Model file for the job. Use its own axes, mm. A direction names the side the tool comes from. Coordinates: 2 decimals unless noted, no trailing zeros. Return JSON: item names as keys, results as strings.
```python
from build123d import *

# Parameters (mm, degrees)
F0_R     = 1
F1_DEPTH = 5
F3_DEPTH = 10.001
F4_R     = 0.3
F6_DEPTH = 2.54
F7_R     = 0.2


with BuildPart() as f1:
    # F0 (on Front) → F1 (new body, symmetric)
    with BuildSketch(Plane.XZ):
        with BuildLine():
            Line((-2, 2), (-2, 0))
            ThreePointArc((-2, 0), (0, -2), (2, 0))
            Line((2, 0), (2, 2))
            Line((2, 2), (0, 2))
            Line((0, 2), (-2, 2))
        make_face()
        Circle(F0_R, mode=Mode.SUBTRACT)
    extrude(amount=F1_DEPTH, both=True)

    # F2 (on face) → F3 (cut, through all)
    with BuildSketch(Plane.XZ.offset(5)):
        with BuildLine():
            Line((0.875, -1.7984368212), (0, 0))
            Line((0, 0), (-0.875, -1.7984368212))
            ThreePointArc((-0.875, -1.7984368212), (0, -2), (0.875, -1.7984368212))
        make_face()
    extrude(amount=-F3_DEPTH, mode=Mode.SUBTRACT)

    # F4
    f4_edges = [f1.edges().sort_by_distance(p)[0] for p in [
        (-0.875, 0, -1.798437),
        (0.875, 0, -1.798437),
        (-1.695582, -5, -1.06066),
        (-2, -5, 1),
        (1.695582, -5, -1.06066),
        (1.695582, 5, -1.06066),
        (2, 5, 1),
        (-1.695582, 5, -1.06066),
        (-2, 5, 1),
        (2, -5, 1),
    ]]
    fillet(f4_edges, radius=F4_R)

    # F5 (on face) → F6 (join)
    with BuildSketch(Plane.XY.offset(2)):
        Polygon((-1.2036230182, 19.6684543043), (-15.6138911843, 19.6684543043), (-15.6138911843, 12.6715609804), (-12.7401659265, 12.6715609804), (-22.5274879485, -2.6133179199), (-25.2762660384, -2.6133179199), (-25.2762660384, -10.0266933441), (-10.8659984544, -10.0266933441), (-10.8659984544, -2.6133179199), (-12.7401659265, -2.6133179199), (-8.4504038095, 4.2169820517), (-6.826125551, 1.676443615), (-8.4504038095, 1.676443615), (-8.4504038095, -5.5286907591), (0, -5.5286907591), (8.4504038095, -5.5286907591), (8.4504038095, 1.676443615), (6.826125551, 1.676443615), (8.4504038095, 4.2169820517), (12.7401659265, -2.6133179199), (10.8659984544, -2.6133179199), (10.8659984544, -10.0266933441), (25.2762660384, -10.0266933441), (25.2762660384, -2.6133179199), (22.5274879485, -2.6133179199), (12.7401659265, 12.6715609804), (15.6138911843, 12.6715609804), (15.6138911843, 19.6684543043), (1.2036230182, 19.6684543043), (1.2036230182, 12.9214497283), (3.6608641967, 12.9214497283), (0, 6.6325762309), (-3.6608641967, 12.9214497283), (-1.2036230182, 12.9214497283), align=None)
        with BuildLine():
            Line((2, 4.7), (2, -4.7))
            ThreePointArc((2, -4.7), (1.9121320344, -4.9121320344), (1.7, -5))
            Line((1.7, -5), (-1.7, -5))
            ThreePointArc((-1.7, -5), (-1.9121320344, -4.9121320344), (-2, -4.7))
            Line((-2, -4.7), (-2, 4.7))
            ThreePointArc((-2, 4.7), (-1.9121320344, 4.9121320344), (-1.7, 5))
            Line((-1.7, 5), (1.7, 5))
            ThreePointArc((1.7, 5), (1.9121320344, 4.9121320344), (2, 4.7))
        make_face(mode=Mode.SUBTRACT)
        with BuildLine():
            ThreePointArc((1.7, -5), (1.9121320344, -4.9121320344), (2, -4.7))
            Line((2, -4.7), (2, 4.7))
            ThreePointArc((2, 4.7), (1.9121320344, 4.9121320344), (1.7, 5))
            Line((1.7, 5), (-1.7, 5))
            ThreePointArc((-1.7, 5), (-1.9121320344, 4.9121320344), (-2, 4.7))
            Line((-2, 4.7), (-2, -4.7))
            ThreePointArc((-2, -4.7), (-1.9121320344, -4.9121320344), (-1.7, -5))
            Line((-1.7, -5), (1.7, -5))
        make_face()
    extrude(amount=F6_DEPTH)

    # F7
    f7_edges = [f1.edges().sort_by_distance(p)[0] for p in [
        (14.177029, 12.671561, 2),
        (17.633827, 5.029122, 2),
        (15.613891, 16.170008, 2),
        (23.901877, -2.613318, 2),
        (8.408757, 19.668454, 2),
        (25.276266, -6.320006, 2),
        (1.203623, 16.294952, 2),
        (18.071132, -10.026693, 2),
        (2.432244, 12.92145, 2),
        (10.865998, -6.320006, 2),
        (1.830432, 9.777013, 2),
        (11.803082, -2.613318, 2),
        (-1.830432, 9.777013, 2),
        (10.595285, 0.801832, 2),
        (-2.432244, 12.92145, 2),
        (7.638265, 2.946713, 2),
        (-1.203623, 16.294952, 2),
        (7.638265, 1.676444, 2),
        (-8.408757, 19.668454, 2),
        (8.450404, -1.926124, 2),
        (-15.613891, 16.170008, 2),
        (0, -5.528691, 2),
        (-14.177029, 12.671561, 2),
        (-8.450404, -1.926124, 2),
        (-17.633827, 5.029122, 2),
        (-7.638265, 1.676444, 2),
        (-23.901877, -2.613318, 2),
        (-7.638265, 2.946713, 2),
        (-25.276266, -6.320006, 2),
        (-10.595285, 0.801832, 2),
        (-18.071132, -10.026693, 2),
        (-11.803082, -2.613318, 2),
        (-10.865998, -6.320006, 2),
        (1.912132, 4.912132, 2),
        (0, 5, 2),
        (-1.912132, 4.912132, 2),
        (-2, 0, 2),
        (-1.912132, -4.912132, 2),
        (0, -5, 2),
        (1.912132, -4.912132, 2),
        (2, 0, 2),
    ]]
    fillet(f7_edges, radius=F7_R)


solid = f1.part
```
Item 1: Drop flat-ended pins along their axis: pin 1 Ø8 at (x, y) = (11.5, -3) entering from -Z; pin 2 Ø1.9 at (y, z) = (15.5, 4) entering from +X; pin 3 Ø0.7 at (y, z) = (-1.5, 3.5) entering from -X; pin 4 Ø2.5 at (y, z) = (-2, 3.5) entering from +X. Give the stop position or say it passes through.
Check result:
{"pin 1": "stops at z = 2", "pin 2": "stops at x = 15.61", "pin 3": "stops at x = -22.04", "pin 4": "stops at x = 25.28"}
Item 2: 3-axis set-ups, long thin cutter, end or side, ignore diameter. For faces 5 (the flat face through (15.614, 16, 3)), 6 (the cylindrical face through (-17.584, 4.995, 2.057)), 7 (the flat face through (-7.65, 2.964, 3.354)), 8 (the flat face through (2, 0, 1)): which of +Z, -Z, +X, -X, +Y, -Y reach the whole face in a straight line?
Check result:
{"face 5": "+Z, -Z, +X, +Y", "face 6": "-Z, -X", "face 7": "+Z, -Z", "face 8": "-Z, +X, +Y, -Y"}
Item 3: Pull direction X, two halves, no side cores. Call faces 1 (the cylindrical face through (1.777, -0.066, -0.918)), 2 (the flat face through (-10.63, 0.75, 3.35)), 3 (the flat face through (-17.565, 5.136, 3.354)), 4 (the cylindrical face through (-10.626, 0.866, 2.057)): +X half, -X half, draft (parallel to the pull), parting line (faces both ways), or undercut.
Check result:
{"face 1": "+X half", "face 2": "undercut", "face 3": "-X half", "face 4": "undercut"}
Item 4: Wall check: line 1 (X direction, y = -2.5, z = 0); line 2 (X direction, y = -8.5, z = 3.75); line 3 (X direction, y = 2.5, z = 1.25). Give the ranges that are in metal, low to high.
Check result:
{"line 1": "x = -2 to -1, 1 to 2", "line 2": "x = -25.28 to -10.87, 10.87 to 25.28", "line 3": "x = -2 to 2"}
Item 5: Saw through at B-B (y = -1.5). Count the separate pieces of the cut face and the enclosed holes in it, and give its area (3 significant figures).
Check result:
{"separate pieces": "3", "enclosed holes": "0", "area": "102 mm2"}
